Check sheet for the modelled part. Datum: model origin and axes. Units: mm. Face numbers are marked on the shaded views. A direction names the side the tool comes from. Round coordinates to 2 decimals unless told otherwise and drop trailing zeros. Write each loop counter-clockwise with the first axis right and the second up, starting at its lowest first coordinate (ties: lowest second). Pieces come first, ordered by that corner, then holes. Notation, with made-up numbers: (48, -4) - (94, -4) arc R19 ccw to (94, 31) - close; hole circle Ø1 at (1.25, 40). An arc over 180 degrees is marked (long way). Answer as a JSON object with one key per item and string values. Group by question number.
Item 1: Sectioned sample at C-C on y = 3.5. Record the boundary of the cut face in (x, z), plus the area to 3 significant figures.
Item 2: Release check for a two-part mould opening along Y. For the marked faces 1, 2, 3 and 4 record: pulls with the +Y half, pulls with the -Y half, needs draft (parallel to the pull), parting line crosses it, or undercut.
Item 3: Sectioned sample at B-B on z = 47. Count the separate pieces of the cut face and the enclosed holes in it, plus the area to 3 significant figures.
Item 4: Gauge pin test, flat ends, axial feed: P1, Ø15, axis at x = 51, y = -36, coming from the +Z side; P2, Ø11.5, axis at x = 24, y = 13, coming from the -Z side; P3, Ø14.5, axis at x = 0, y = 36, coming from the +Z side. Record the tip position at first contact, or that the pin passes through.
Item 5: Sectioned sample at A-A on z = 12.5. Record the boundary of the cut face in (x, y).
Item 6: Thickness scan on line 1 (Y direction, x = 0, z = 45); line 2 (Y direction, x = 20, z = 53); line 3 (Z direction, x = 65.5, y = 20). Record the ranges inside material, lowest first.
Item 7: Set-up check for the marked faces 5, 6 and 7: record each of +Z, -Z, +X, -X, +Y, -Y from which the full face is reachable in a straight line by a thin tool's end or side.
Item 8: Sectioned sample at D-D on x = 35. Record the boundary of the cut face in (y, z).
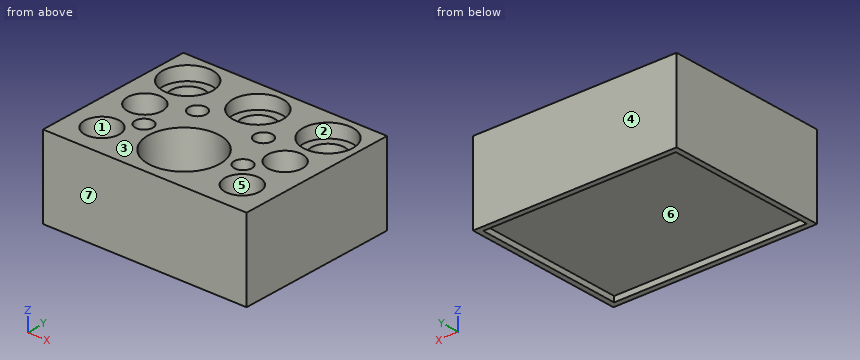
```python
from build123d import *

# Parameters (mm, degrees)
F0_W      = 148
F0_H      = 118
F1_DEPTH  = 59
F2_R      = 14
F3_DEPTH  = 50.5
F2_R_2    = 25.75
F4_DEPTH  = 28
F2_R_3    = 12
F5_DEPTH  = 21.5
F2_R_4    = 18
F6_DEPTH  = 10
F2_R_5    = 6.4
F7_DEPTH  = 8.5
F2_R_6    = 12.5
F8_DEPTH  = 20
F9_W      = 140
F9_H      = 110
F10_DEPTH = 4


with BuildPart() as f1:
    # F0 (on Top) → F1 (new body)
    with BuildSketch(Plane.XY):
        Rectangle(F0_W, F0_H)
    extrude(amount=F1_DEPTH)

    # F2 (on face) → F3 (cut)
    with BuildSketch(Plane.XY.offset(59)):
        with Locations((0, -26)):
            Circle(F2_R)
    extrude(amount=-F3_DEPTH, mode=Mode.SUBTRACT)

    # F2 (on face) → F4 (cut)
    with BuildSketch(Plane.XY.offset(59)):
        with Locations((0, -26)):
            Circle(F2_R_2)
        with Locations((0, -26)):
            Circle(F2_R, mode=Mode.SUBTRACT)
    extrude(amount=-F4_DEPTH, mode=Mode.SUBTRACT)

    # F2 (on face) → F5 (cut)
    with BuildSketch(Plane.XY.offset(59)):
        with Locations((-51, 36)):
            Circle(F2_R_3)
        with Locations((0, 36)):
            Circle(F2_R_3)
        with Locations((51, 36)):
            Circle(F2_R_3)
    extrude(amount=-F5_DEPTH, mode=Mode.SUBTRACT)

    # F2 (on face) → F6 (cut)
    with BuildSketch(Plane.XY.offset(59)):
        with Locations((-51, 36)):
            Circle(F2_R_4)
        with Locations((-51, 36)):
            Circle(F2_R_3, mode=Mode.SUBTRACT)
        with Locations((0, 36)):
            Circle(F2_R_4)
        with Locations((0, 36)):
            Circle(F2_R_3, mode=Mode.SUBTRACT)
        with Locations((51, 36)):
            Circle(F2_R_4)
        with Locations((51, 36)):
            Circle(F2_R_3, mode=Mode.SUBTRACT)
    extrude(amount=-F6_DEPTH, mode=Mode.SUBTRACT)

    # F2 (on face) → F7 (cut)
    with BuildSketch(Plane.XY.offset(59)):
        with Locations((-36, -18)):
            Circle(F2_R_5)
        with Locations((-24, 13)):
            Circle(F2_R_5)
        with Locations((24, 13)):
            Circle(F2_R_5)
        with Locations((36, -18)):
            Circle(F2_R_5)
    extrude(amount=-F7_DEPTH, mode=Mode.SUBTRACT)

    # F2 (on face) → F8 (cut)
    with BuildSketch(Plane.XY.offset(59)):
        with Locations((-51, -36)):
            Circle(F2_R_6)
        with Locations((-51, 0)):
            Circle(F2_R_6)
        with Locations((51, 0)):
            Circle(F2_R_6)
        with Locations((51, -36)):
            Circle(F2_R_6)
    extrude(amount=-F8_DEPTH, mode=Mode.SUBTRACT)

    # F9 (on face) → F10 (cut)
    with BuildSketch(Plane.XY):
        Rectangle(F9_W, F9_H)
    extrude(amount=F10_DEPTH, mode=Mode.SUBTRACT)


solid = f1.part
```
Completed:
{
 "1": {"outline": "(-74, 0) - (-70, 0) - (-70, 4) - (70, 4) - (70, 0) - (74, 0) - (74, 59) - (63, 59) - (63, 39) - (39, 39) - (39, 59) - (-39, 59) - (-39, 39) - (-63, 39) - (-63, 59) - (-74, 59) - close", "area": "7,210 mm²"},
 "2": {"face 1": "undercut", "face 2": "undercut", "face 3": "needs draft", "face 4": "pulls with the +Y half"},
 "3": {"separate pieces": "1", "enclosed holes": "8", "area": "12,100 mm²"},
 "4": {"P1": "z = 39", "P2": "z = 4", "P3": "z = 37.5"},
 "5": {"outline": "(-74, -59) - (74, -59) - (74, 59) - (-74, 59) - close; hole circle Ø28 at (0, -26)"},
 "6": {"line 1": "-59 to -51.75, -0.25 to 24, 48 to 59", "line 2": "-59 to -42.22, -9.78 to 8, 18 to 59", "line 3": "4 to 59"},
 "7": {"face 5": "+Z", "face 6": "-Z", "face 7": "+Z, -Z, +X, -X, -Y"},
 "8": {"outline": "(-59, 0) - (-55, 0) - (-55, 4) - (55, 4) - (55, 0) - (59, 0) - (59, 59) - (44.25, 59) - (44.25, 49) - (27.75, 49) - (27.75, 59) - (-11.68, 59) - (-11.68, 50.5) - (-24.32, 50.5) - (-24.32, 59) - (-59, 59) - close"}
}
